The figure shows three views and two pictorial views of one solid part (mm, origin at its lowest corner). Answer the questions. Coordinates: 2 decimals unless noted, no trailing zeros. Order: outer loops, then holes, each group sorted by start corner. A loop starts at its lowest first (then second) coordinate and runs counter-clockwise, first axis right, second up. Notation, with made-up numbers: (71, 46.5) -> (91, 46.5) arc R35 cw to (91, 79.5) -> close; hole circle Ø7 at (-36, 75.5). An arc over 180 degrees is marked (long way). Write item = value, one per line. Start each with the question number.
Q1. Flat-ended cylindrical pins translate along their axes: pin 1 (11.5 mm diameter, centred on x = 60, y = 110.21, fed in from -Z); pin 2 (1.5 mm diameter, centred on y = 33.5, z = 25.5, fed in from -X); pin 3 (10 mm diameter, centred on y = 79.5, z = 34, fed in from +X); pin 4 (4 mm diameter, centred on x = 50, z = 8.5, fed in from +Y). Find the tip coordinate at first contact, or state that the pin passes through.
Q2. The part is cut by section C-C, the plane x = 107.75. Determine the outline of the cut face in (y, z) (1 decimal), plus the area to 3 significant figures.
Q3. The part is cut by section A-A, the plane x = 60. Determine the outline of the cut face in (y, z), plus the area to 3 significant figures.
Q4. For a pull along Y with two mould halves and no side action, classify the marked faces 1, 2 and 3 as +Y half, -Y half, draft (parallel to the pull), parting line (faces both ways), or undercut.
Q5. Straight lines are drawn through the part: L1, parallel to Y at x = 60, z = 31; L2, parallel to Y at x = 59, z = 25.5 (1 decimal); L3, parallel to X at y = 29.5, z = 46. For each, find the intervals that lie inside material, in ascending order. Write a range as from..to.
Q6. The part is cut by section D-D, the plane z = 19.5. Count the separate pieces of the cut face and the enclosed holes in it.
Q7. The part is cut by section B-B, the plane y = 41.5. Determine the outline of the cut face in (x, z) (1 decimal), plus the area to 3 significant figures.
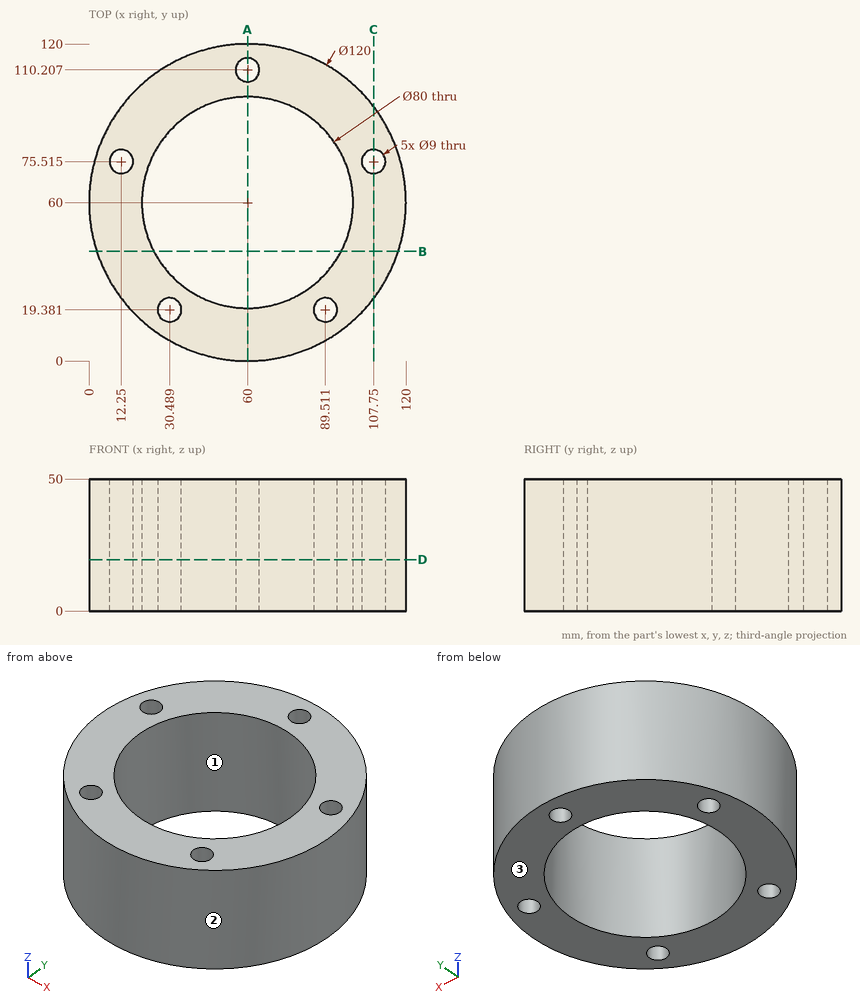
Model answer:
q1.pin_1 = 0
q1.pin_2 = 5.81
q1.pin_3 = 118.22
q1.pin_4 = 119.46
q2.outline = (23.7, 0) -> (71, 0) -> (71, 50) -> (23.7, 50) -> close; (80, 0) -> (96.3, 0) -> (96.3, 50) -> (80, 50) -> close
q2.area = 3,180 mm2
q3.outline = (0, 0) -> (20, 0) -> (20, 50) -> (0, 50) -> close; (100, 0) -> (105.71, 0) -> (105.71, 50) -> (100, 50) -> close; (114.71, 0) -> (120, 0) -> (120, 50) -> (114.71, 50) -> close
q3.area = 1,550 mm2
q4.face_1 = undercut
q4.face_2 = parting line
q4.face_3 = draft
q5.L1 = 0..20, 100..105.71, 114.71..120
q5.L2 = 0..20, 100..105.8, 114.6..120
q5.L3 = 8.33..34.12, 85.88..111.67
q6.separate_pieces = 1
q6.enclosed_holes = 6
q7.outline = (2.9, 0) -> (24.5, 0) -> (24.5, 50) -> (2.9, 50) -> close; (95.5, 0) -> (117.1, 0) -> (117.1, 50) -> (95.5, 50) -> close
q7.area = 2,160 mm2
